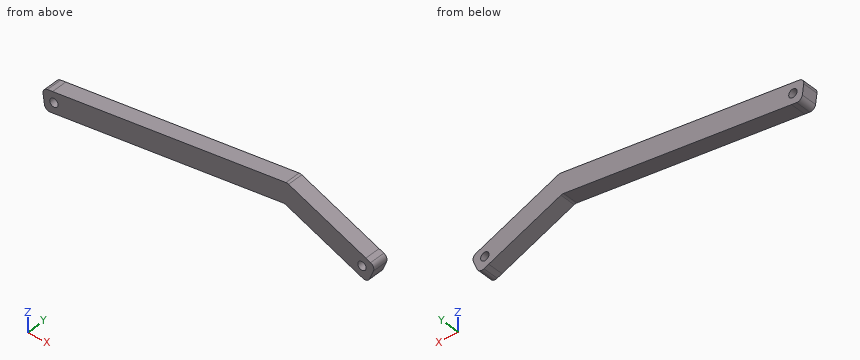
Autodesk Inventor part; units mm, degrees
ref_plane "YZ Plane" through (0, 0, 0) normal (1, 0, 0) x (0, 1, 0)
ref_plane "XZ Plane" through (0, 0, 0) normal (0, 1, 0) x (-1, 0, 0)
ref_plane "XY Plane" through (0, 0, 0) normal (0, 0, 1) x (1, 0, 0)
sketch "Sketch1" plane through (0, 0, 0) normal (0, 1, 0) x (-1, 0, 0)
  line L0 (0, 0) -> (190.5, 0)
  line L1 (190.5, 0) -> (47.0141, 19.3142)
  line L2 (47.0141, 19.3142) -> (0, 0)
  line L3 (2.413, -5.8737) -> (-2.413, 5.8737)
  line L4 (-2.413, 5.8737) -> (45.388, 25.5111)
  line L5 (47.0663, 12.4707) -> (2.413, -5.8737)
  line L6 (41.2492, 26.4974) -> (39.555, 13.9109)
  line L7 (48.6964, 12.6805) -> (189.6529, -6.2932)
  line L8 (189.6529, -6.2932) -> (191.3471, 6.2932)
  line L9 (191.3471, 6.2932) -> (47.0181, 25.7209)
  arc A0 (47.0181, 25.7209) -> (45.388, 25.5111) centre (46.5945, 22.5743) ccw
  arc A1 (48.6964, 12.6805) -> (47.0663, 12.4707) centre (48.2728, 9.5338) ccw
  circle A2 centre (47.0141, 19.3142) radius 2.5797
  circle A3 centre (190.5, 0) radius 2.5797
  circle A4 centre (0, 0) radius 2.5797
  line L10 (191.3471, 6.2932) -> (189.6529, -6.2932)
  line L11 (189.6529, -6.2932) -> (192.7995, -6.7168)
  line L12 (196.3697, -3.9937) -> (197.2168, 2.2995)
  line L13 (194.4937, 5.8697) -> (191.3471, 6.2932)
  arc A5 (197.2168, 2.2995) -> (194.4937, 5.8697) centre (194.0702, 2.7231) ccw
  arc A6 (192.7995, -6.7168) -> (196.3697, -3.9937) centre (193.2231, -3.5702) ccw
  line L14 (-2.413, 5.8737) -> (2.413, -5.8737)
  line L15 (2.413, -5.8737) -> (-0.5238, -7.0802)
  line L16 (-4.6672, -5.3498) -> (-7.0802, 0.5238)
  line L17 (-5.3498, 4.6672) -> (-2.413, 5.8737)
  arc A7 (-5.3498, 4.6672) -> (-7.0802, 0.5238) centre (-4.1433, 1.7303) ccw
  arc A8 (-4.6672, -5.3498) -> (-0.5238, -7.0802) centre (-1.7303, -4.1433) ccw
  point P0 (195.9461, -7.1404)
  point P1 (-3.4607, -8.2867)
  dimension "d0" = 190.5
  dimension "d1" = 150
  dimension "d2" = 12.7
  dimension "d3" = 3.175
  dimension "d4" = 5.1594
  dimension "d6" = 6.35
  dimension "d7" = 3.175
  dimension "d8" = 6.35
  dimension "d9" = 3.175
  dimension "d12" = 144.78
  dimension "d13" = 12.7
  dimension "d14" = 12.7
extrude "Extrusion1" add sketch "Sketch1" along normal blind 9.525 contours A4 L2 A2 L1 A3 L0 L7 A1 L5 | L0 L5 L3 A4 | A4 L3 L4 L6 L2 | L3 L15 A8 L16 A7 L17 A4 | L6 L4 A0 L9 L8 A3 L1 A2 L2 | L0 A3 L8 L7 | A2 L1 L2 | L2 L1 A2 | L8 A3 L13 A5 L12 A6 L11
Geometry: final body of the model. Coordinates: model frame, mm. Coordinates: 2 decimals unless noted, no trailing zeros. Loops run counter-clockwise (first coordinate to the right, second up) from the corner with the lowest first, then second, coordinate; pieces in that order, holes last. Notation, with made-up numbers: (21, 77) -> (63, 77) arc R15 ccw to (63, 97) -> close; hole circle Ø3 at (55.25, 64.5). An arc over 180 degrees is marked (long way). Use a Markdown table: item, result. Add a question column.
(1) Line query: line 1 along Z through (x, y) = (0, 7) (3 decimals); line 2 along Z through (x, y) = (-190.5, 2); line 3 along Z through (x, y) = (-160.5, 8.5). Output: solid intervals per line, ascending.
(2) Section query C-C, the plane x = -172.5. Return loops of the section in (y, z) (3 decimals), plus the area to 3 significant figures.
(3) Section query A-A, the plane y = 6. Return loops of the section in (x, z), plus the area to 3 significant figures.
(4) Section query B-B, the plane z = 21. Return loops of the section in (x, y) (3 decimals).
(5) Pin query (flat end, axial travel): pin 1 Ø3 at (x, y) = (-91.5, 5.5) entering from +Z; pin 2 Ø1 at (x, y) = (-90.5, 5) entering from -Z; pin 3 Ø3 at (x, y) = (-129.5, 1) entering from -Z. Return the tip coordinate at first contact, or that it passes through.
Answer:
| question | item | result |
|---|---|---|
| 1 | line 1 | z = -6.865 to -2.58, 2.58 to 6.865 |
| 1 | line 2 | z = -6.41 to -2.58, 2.58 to 6.41 |
| 1 | line 3 | z = -2.37 to 10.45 |
| 2 | outline | (0, -3.984) -> (9.525, -3.984) -> (9.525, 8.83) -> (0, 8.83) -> close |
| 2 | area | 122 mm^2 |
| 3 | outline | (-197.22, 2.3) -> (-196.37, -3.99) arc R3.17 ccw to (-192.8, -6.72) -> (-189.65, -6.29) -> (-48.7, 12.68) arc R3.17 cw to (-47.07, 12.47) -> (-2.41, -5.87) -> (0.52, -7.08) arc R3.18 ccw to (4.67, -5.35) -> (7.08, 0.52) arc R3.18 ccw to (5.35, 4.67) -> (2.41, 5.87) -> (-45.39, 25.51) arc R3.17 ccw to (-47.02, 25.72) -> (-191.35, 6.29) -> (-194.49, 5.87) arc R3.17 ccw to start; hole circle Ø5.16 at (-190.5, 0); hole circle Ø5.16 at (0, 0) |
| 3 | area | 2,600 mm^2 |
| 4 | outline | (-82.09, 0) -> (-34.407, 0) -> (-34.407, 9.525) -> (-82.09, 9.525) -> close |
| 5 | pin 1 | stops at z = 19.94 |
| 5 | pin 2 | stops at z = 6.99 |
| 5 | pin 3 | stops at z = 1.6 |
